from build123d import *

# Parameters (mm, degrees)
F1_DEPTH = 3
F2_SIZE  = 0.5


with BuildPart() as f1:
    # F0 (on Top) → F1 (new body)
    with BuildSketch(Plane.XY):
        Polygon((6, 23.656854), (8.843146, 26.5), (21.35, 26.5), (21.35, 29.5), (6, 29.5), (6, 32.5), (3, 32.5), (3, 29.5), (0, 29.5), (0, 26.5), (3, 26.5), (3, 18.5), (0, 18.5), (0, 15.5), (3, 15.5), (3, 0), (6, 0), (6, 15.5), (21.35, 15.5), (21.35, 18.5), (8.843146, 18.5), (6, 21.343146), align=None)
    extrude(amount=F1_DEPTH)

    # F2
    f2_edges = [f1.edges().sort_by_distance(p)[0] for p in [
        (0, 29.5, 1.5),
        (0, 26.5, 1.5),
        (0, 18.5, 1.5),
        (0, 15.5, 1.5),
        (21.35, 15.5, 1.5),
        (21.35, 26.5, 1.5),
        (3, 32.5, 1.5),
        (6, 32.5, 1.5),
        (21.35, 29.5, 1.5),
        (21.35, 18.5, 1.5),
        (6, 15.5, 1.5),
        (6, 29.5, 1.5),
    ]]
    chamfer(f2_edges, length=F2_SIZE)

    # F3: F1 across face


with BuildPart() as f1_1:
    add(f1.part)
    add(f1.part.mirror(Plane(origin=(4.5, 0, 1.5), x_dir=(1, 0, 0), z_dir=(0, -1, 0))))


solid = f1_1.part
Verification items for the finished model (mm, model axes). A direction names the side the tool comes from. Coordinates: 2 decimals unless noted, no trailing zeros. Order: outer loops, then holes, each group sorted by start corner. A loop starts at its lowest first (then second) coordinate and runs counter-clockwise, first axis right, second up. Notation, with made-up numbers: M 27,66.25 L 75,66.25 A19 cw 75,71.25 Z; hole C 87,75.5 d2. An arc over 180 degrees is marked long. One line per item, written item: value. Start each with the question number.
Item 1: Sectioned sample at B-B (y = 3). Enter the section's corners in (x, z), then the cut area to 3 significant figures.
Item 2: Scan lines: probe 1 along Y at (x, z) = (14.75, 1.3); probe 2 along Y at (x, z) = (8.5, 1.45); probe 3 along X at (y, z) = (23, 2.15). Record each from-to range of solid material in increasing order.
Item 3: Gauge pin test, flat ends, axial feed: pin 1 (0.8 mm diameter, centred on x = 2, z = 2, fed in from -Y); pin 2 (1.5 mm diameter, centred on y = -2, z = 2, fed in from -X); pin 3 (1.5 mm diameter, centred on y = 5, z = 2, fed in from +X); pin 4 (6 mm diameter, centred on x = 17.5, y = 10.5, fed in from +Z). Record the tip position at first contact, or that the pin passes through.
Item 4: Sectioned sample at A-A (x = 16.75). Enter the section's corners in (y, z).
Item 5: Access from +Z, -Z, +X, -X, +Y, -Y to the whole of each face (thin tool, end or side, straight path). Record for faces 1 (the flat face through (6, -31, 1)), 2 (the flat face through (2, -29.5, 1)), 3 (the flat face through (6, 31, 1)), 4 (the flat face through (15, 26.5, 1)).
Item 6: Sectioned sample at C-C (x = 7.25). Enter the section's corners in (y, z), then the cut area to 3 significant figures.
Conclusion:
1. outline: M 3,0 L 6,0 L 6,3 L 3,3 Z
1. area: 9.00 mm^2
2. probe 1: y = -29.5 to -26.5, -18.5 to -15.5, 15.5 to 18.5, 26.5 to 29.5
2. probe 2: y = -29.5 to -26.16, -18.84 to -15.5, 15.5 to 18.84, 26.16 to 29.5
2. probe 3: x = 3 to 6
3. pin 1: stops at y = -29.5
3. pin 2: stops at x = 3
3. pin 3: stops at x = 6
3. pin 4: passes through
4. outline: M -29.5,0 L -26.5,0 L -26.5,3 L -29.5,3 Z; M -18.5,0 L -15.5,0 L -15.5,3 L -18.5,3 Z; M 15.5,0 L 18.5,0 L 18.5,3 L 15.5,3 Z; M 26.5,0 L 29.5,0 L 29.5,3 L 26.5,3 Z
5. face 1: +Z, -Z, +X, -Y
5. face 2: +Z, -Z, -X, -Y
5. face 3: +Z, -Z, +X, +Y
5. face 4: +Z, -Z, +X
6. outline: M -29.5,0 L -24.91,0 L -24.91,3 L -29.5,3 Z; M -20.09,0 L -15.5,0 L -15.5,3 L -20.09,3 Z; M 15.5,0 L 20.09,0 L 20.09,3 L 15.5,3 Z; M 24.91,0 L 29.5,0 L 29.5,3 L 24.91,3 Z
6. area: 55.1 mm^2
